Geometry check sheet. Reference: the model listing, model coordinates, mm. Give positions to 0.01 mm unless a question says otherwise; leave off trailing zeros. Loops run counter-clockwise (first coordinate to the right, second up) from the corner with the lowest first, then second, coordinate; pieces in that order, holes last. Notation, with made-up numbers: (72, 10.25) - (108, 10.25) arc R23 ccw to (108, 44.25) - close; hole circle Ø8 at (73, 9). An arc over 180 degrees is marked (long way). One line per question, with ' | ' between items. Start each with the question number.
from build123d import *

# Parameters (mm, degrees)
SKETCH_1_W               = 16
SKETCH_1_H               = 16
EXTRUDE_1_DEPTH          = 12
SKETCH_2_R               = 3
CUT_EXTRUDE_2_DEPTH      = 17.492422502
SKETCH_3_R               = 1.25
CUT_EXTRUDE_3_DEPTH      = 22.540659229
SKETCH_4_R               = 3
CUT_EXTRUDE_4_DEPTH      = 22.540659229
CHAMFER_1_SIZE           = 0.5
CUT_EXTRUDE_5_REACH      = 18.492
CUT_EXTRUDE_5_END_RADIUS = 3
SKETCH_5_R               = 1.5


with BuildPart() as part:
    # 草圖1 → 填料-伸長1 (new body)
    with BuildSketch(Plane(origin=(0, 0, 0), x_dir=(1, 0, 0), z_dir=(0, 1, 0))):
        Rectangle(SKETCH_1_W, SKETCH_1_H)
    extrude(amount=EXTRUDE_1_DEPTH)

    # 草圖2 → 除料-伸長2 (cut, through all)
    with BuildSketch(Plane(origin=(0, 12, 0), x_dir=(1, 0, 0), z_dir=(0, 1, 0))):
        with Locations(Location((-4.5, 0, 0), (0, 0, 270))):
            Circle(SKETCH_2_R)
    extrude(amount=-CUT_EXTRUDE_2_DEPTH, mode=Mode.SUBTRACT)

    # 草圖3 → 除料-伸長3 (cut, through all)
    with BuildSketch(Plane.XY.offset(8)):
        with Locations((5.25, 1.75)):
            Circle(SKETCH_3_R)
    extrude(amount=-CUT_EXTRUDE_3_DEPTH, mode=Mode.SUBTRACT)

    # 草圖4 → 除料-伸長4 (cut, through all)
    with BuildSketch(Plane.XY.offset(8)):
        with Locations((3, 7)):
            Circle(SKETCH_4_R)
    extrude(amount=-CUT_EXTRUDE_4_DEPTH, mode=Mode.SUBTRACT)

    # 導角1
    chamfer_1_edges = [part.edges().sort_by_distance(p)[0] for p in [
        (8, 12, 0),
        (0, 12, -8),
        (-8, 12, 0),
        (0, 0, -8),
        (8, 0, 0),
        (0, 0, 8),
        (-8, 0, 0),
        (0, 12, 8),
        (-8, 6, -8),
        (8, 6, -8),
        (8, 6, 8),
        (-8, 6, 8),
    ]]
    chamfer(chamfer_1_edges, length=CHAMFER_1_SIZE - 0.0001)  # a hair under: the kernel refuses the full size

    # 除料-伸長5: up to this cylinder (the profile starts outside it)
    cut_extrude_5_end = Plane(origin=(3, 7, 0), z_dir=(0, 0, 1)) * Cylinder(CUT_EXTRUDE_5_END_RADIUS, 43.984, mode=Mode.PRIVATE)
    # 草圖5 → 除料-伸長5 (cut, up to the surface)
    with BuildSketch(Plane(origin=(0, 12, 0), x_dir=(1, 0, 0), z_dir=(0, 1, 0)), mode=Mode.PRIVATE) as cut_extrude_5_sk1:
        with Locations(Location((3, 0, 0), (0, 0, 270))):
            Circle(SKETCH_5_R)
    cut_extrude_5_tool1 = extrude(cut_extrude_5_sk1.sketch, amount=-CUT_EXTRUDE_5_REACH, mode=Mode.PRIVATE) - cut_extrude_5_end
    add(cut_extrude_5_tool1.solids().sort_by_distance((3, 12, 0))[0], mode=Mode.SUBTRACT)


solid = part.part
(1) Section check B-B, the plane z = 0. Count the separate pieces of the cut face and the enclosed holes in it, and give its area (3 significant figures).
(2) Material ranges on line 1 (X direction, y = 10.2, z = 0); line 2 (X direction, y = 6.75, z = -0.5); line 3 (Y direction, x = 3, z = -2.5), recorded low to high.
(3) Section check A-A, the plane y = 1.75. Record the boundary of the cut face in (x, z).
(4) Mould release check, pull along Z, two halves, no side actions. Record for faces 1 (the face through (2.425, 10.816, 1.386)), 2 (the face through (-2, 6, 8)), 3 (the face through (-2, 6, -8)), 4 (the face through (-8, 6, 0)): pulls with the +Z half, pulls with the -Z half, needs draft (parallel to the pull), parting line crosses it, or undercut.
(5) Section check D-D, the plane x = -4.5. Record the boundary of the cut face in (y, z).
(6) Section check C-C, the plane x = 3. Record the boundary of the cut face in (y, z).
Numbers:
1) separate pieces: 2 | enclosed holes: 1 | area: 79.9 mm^2
2) line 1: -8 to -7.5, -1.5 to 1.5, 4.5 to 8 | line 2: -8 to -7.46, -1.54 to 0.01, 5.99 to 8 | line 3: 0 to 4, 10 to 12
3) outline: (-8, -7.5) - (-7.5, -8) - (4, -8) - (4, 8) - (-7.5, 8) - (-8, 7.5) - close; (6.5, -8) - (7.5, -8) - (8, -7.5) - (8, 7.5) - (7.5, 8) - (6.5, 8) - close; hole circle Ø6 at (-4.5, 0)
4) face 1: undercut | face 2: pulls with the +Z half | face 3: pulls with the -Z half | face 4: needs draft
5) outline: (0, -7.5) - (0.5, -8) - (11.5, -8) - (12, -7.5) - (12, -3) - (0, -3) - close; (0, 3) - (12, 3) - (12, 7.5) - (11.5, 8) - (0.5, 8) - (0, 7.5) - close
6) outline: (0, -7.5) - (0.5, -8) - (4, -8) - (4, 8) - (0.5, 8) - (0, 7.5) - close; (10, -8) - (11.5, -8) - (12, -7.5) - (12, -1.5) - (10, -1.5) - close; (10, 1.5) - (12, 1.5) - (12, 7.5) - (11.5, 8) - (10, 8) - close
